Source: CAD feature listing. Evaluate the final solid. Frame: model axes, mm. Face numbers are marked on the shaded views. A direction names the side the tool comes from. Round coordinates to 2 decimals unless told otherwise and drop trailing zeros. Loops run counter-clockwise (first coordinate to the right, second up) from the corner with the lowest first, then second, coordinate; pieces in that order, holes last. Notation, with made-up numbers: M -25.5,17.5 L -16.5,17.5 A13 cw -16.5,23.5 Z; hole C 77.25,83 d10. An arc over 180 degrees is marked long. Answer as a JSON object with one key per item and string values.
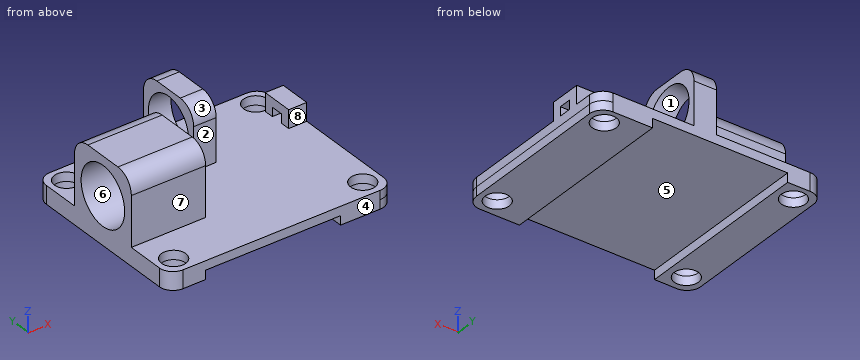
from build123d import *

# Parameters (mm, degrees)
CROQUIS1_W               = 49.8
CROQUIS1_H               = 39.8
CROQUIS1_R               = 2.7
SALIENTE_EXTRUIR1_DEPTH  = 6
CORTAR_EXTRUIR1_DEPTH    = 4
SALIENTE_EXTRUIR3_DEPTH  = 3
CROQUIS5_R               = 6.35
CORTAR_EXTRUIR2_DEPTH    = 3
SALIENTE_EXTRUIR4_DEPTH  = 10
SALIENTE_EXTRUIR5_DEPTH  = 2
CORTAR_EXTRUIR3_START    = -3
CORTAR_EXTRUIR3_DEPTH    = 3
CORTAR_EXTRUIR4_DEPTH    = 4
CROQUIS10_W              = 4
CROQUIS10_H              = 7
SALIENTE_EXTRUIR6_DEPTH  = 4
CORTAR_EXTRUIR5_START    = -4
CORTAR_EXTRUIR5_DEPTH    = 4
CROQUIS16_W              = 28.958796265
CROQUIS16_H              = 47.870649268
CORTAR_EXTRUIR6_DEPTH    = 2
CROQUIS17_W              = 5
CROQUIS17_H              = 16
CORTAR_EXTRUIR7_DEPTH    = 10
CORTAR_EXTRUIR8_DEPTH    = 2
SALIENTE_EXTRUIR7_DEPTH  = 2
CROQUIS22_R              = 6.5
SALIENTE_EXTRUIR9_DEPTH  = 15
SALIENTE_EXTRUIR10_DEPTH = 1.5
CROQUIS25_W              = 5
CROQUIS25_H              = 15
SALIENTE_EXTRUIR11_DEPTH = 13.5
CORTAR_EXTRUIR9_START    = -5
CROQUIS26_R              = 6
CORTAR_EXTRUIR9_DEPTH    = 5
REDONDEO2_R              = 4
CROQUIS27_W              = 8
CROQUIS27_H              = 39.8
CROQUIS27_R              = 2.7
CROQUIS27_W_2            = 11.8
SALIENTE_EXTRUIR13_DEPTH = 2
REDONDEO3_R              = 3


with BuildPart() as part:
    # Croquis1 → Saliente-Extruir1 (new body)
    with BuildSketch(Plane.XY):
        with Locations((-31.963412372, -3.757931034)):
            Rectangle(CROQUIS1_W, CROQUIS1_H)
        with Locations((-52.963412372, 12.342068966)):
            Circle(CROQUIS1_R, mode=Mode.SUBTRACT)
        with Locations((-10.963412372, 12.342068966)):
            Circle(CROQUIS1_R, mode=Mode.SUBTRACT)
        with Locations((-10.963412372, -19.657931034)):
            Circle(CROQUIS1_R, mode=Mode.SUBTRACT)
        with Locations((-52.963412372, -19.657931034)):
            Circle(CROQUIS1_R, mode=Mode.SUBTRACT)
    extrude(amount=SALIENTE_EXTRUIR1_DEPTH)

    # Croquis2 → Cortar-Extruir1 (cut)
    with BuildSketch(Plane.XY.offset(6)):
        with BuildLine():
            Line((-49.963412372, -16.757931034), (-13.963412372, -16.757931034))
            ThreePointArc((-13.963412372, -16.757931034), (-12.54919881, -16.172144597), (-11.963412372, -14.757931034))
            Line((-11.963412372, -14.757931034), (-11.963412372, 7.242068966))
            ThreePointArc((-11.963412372, 7.242068966), (-12.54919881, 8.656282528), (-13.963412372, 9.242068966))
            Line((-13.963412372, 9.242068966), (-49.963412372, 9.242068966))
            ThreePointArc((-49.963412372, 9.242068966), (-51.377625934, 8.656282528), (-51.963412372, 7.242068966))
            Line((-51.963412372, 7.242068966), (-51.963412372, -14.757931034))
            ThreePointArc((-51.963412372, -14.757931034), (-51.377625934, -16.172144597), (-49.963412372, -16.757931034))
        make_face()
    extrude(amount=-CORTAR_EXTRUIR1_DEPTH, mode=Mode.SUBTRACT)

    # Croquis4 → Saliente-Extruir3 (add)
    with BuildSketch(Plane(origin=(0, 0, 0), x_dir=(-1, 0, 0), z_dir=(0, 0, -1))):
        with BuildLine():
            Line((56.863412372, 4.242068966), (61.863412372, 4.242068966))
            Line((61.863412372, 4.242068966), (61.863412372, -0.257931034))
            Line((61.863412372, -0.257931034), (57.863412372, -0.257931034))
            ThreePointArc((57.863412372, -0.257931034), (57.358118834, -0.294597605), (56.863412372, -0.403829068))
            Line((56.863412372, -0.403829068), (56.863412372, 4.242068966))
        make_face()
        with BuildLine():
            Line((61.863412372, -11.757931034), (56.863412372, -11.757931034))
            Line((56.863412372, -11.757931034), (56.863412372, -7.112033001))
            ThreePointArc((56.863412372, -7.112033001), (57.358118834, -7.221264464), (57.863412372, -7.257931034))
            Line((57.863412372, -7.257931034), (61.863412372, -7.257931034))
            Line((61.863412372, -7.257931034), (61.863412372, -11.757931034))
        make_face()
    extrude(amount=-SALIENTE_EXTRUIR3_DEPTH)

    # Croquis5 → Cortar-Extruir2 (cut)
    with BuildSketch(Plane.XY.offset(3)):
        with Locations((-57.863412372, -3.757931034)):
            Circle(CROQUIS5_R)
    extrude(amount=CORTAR_EXTRUIR2_DEPTH, mode=Mode.SUBTRACT)

    # Croquis6 → Saliente-Extruir4 (add)
    with BuildSketch(Plane.XY.offset(3)):
        with BuildLine():
            Line((-61.863412372, 4.242068966), (-51.963412372, 4.242068966))
            Line((-51.963412372, 4.242068966), (-48.963412372, 4.242068966))
            Line((-48.963412372, 4.242068966), (-48.963412372, -11.757931034))
            Line((-48.963412372, -11.757931034), (-51.963412372, -11.757931034))
            Line((-51.963412372, -11.757931034), (-61.863412372, -11.757931034))
            Line((-61.863412372, -11.757931034), (-61.863412372, -8.689715701))
            ThreePointArc((-61.863412372, -8.689715701), (-51.513412372, -3.757931034), (-61.863412372, 1.173853632))
            Line((-61.863412372, 1.173853632), (-61.863412372, 4.242068966))
        make_face()
    extrude(amount=SALIENTE_EXTRUIR4_DEPTH)

    # Croquis7 → Saliente-Extruir5 (add)
    with BuildSketch(Plane.XY.offset(2)):
        Polygon((-51.963412372, -3.757931034), (-51.963412372, 4.242068966), (-48.963412372, 4.242068966), (-48.963412372, -11.757931034), (-51.963412372, -11.757931034), align=None)
    extrude(amount=SALIENTE_EXTRUIR5_DEPTH)

    # Croquis8 → Cortar-Extruir3 (cut)
    with BuildSketch(Plane.XY.offset(3).offset(CORTAR_EXTRUIR3_START)):
        with BuildLine():
            Line((-56.863412372, -0.403829068), (-56.863412372, -7.112033001))
            ThreePointArc((-56.863412372, -7.112033001), (-53.509310406, -3.757931034), (-56.863412372, -0.403829068))
        make_face()
    extrude(amount=CORTAR_EXTRUIR3_DEPTH, mode=Mode.SUBTRACT)

    # Croquis9 → Cortar-Extruir4 (cut)
    with BuildSketch(Plane.XY.offset(6)):
        Polygon((-56.863412372, -11.757931034), (-56.863412372, -27.492217147), (-1.817084798, -27.492217147), (-1.817084798, 22.861833321), (-56.863412372, 22.861833321), (-56.863412372, 4.242068966), (-47.172737702, 4.242068966), (-47.172737702, -11.757931034), align=None)
    extrude(amount=-CORTAR_EXTRUIR4_DEPTH, mode=Mode.SUBTRACT)

    # Croquis10 → Saliente-Extruir6 (add)
    with BuildSketch(Plane.XY.offset(2)):
        with Locations((-9.063412372, 5.842068966)):
            Rectangle(CROQUIS10_W, CROQUIS10_H)
    extrude(amount=SALIENTE_EXTRUIR6_DEPTH)

    # Croquis11 → Cortar-Extruir5 (cut)
    with BuildSketch(Plane(origin=(-7.063412372, 0, 0), x_dir=(0, 0, -1), z_dir=(1, 0, 0)).offset(CORTAR_EXTRUIR5_START)):
        Polygon((-2, 5.842068966), (-2, 7.242068966), (-4, 7.242068966), (-4, 4.442068966), (-2, 4.442068966), align=None)
    extrude(amount=CORTAR_EXTRUIR5_DEPTH, mode=Mode.SUBTRACT)

    # Croquis16 → Cortar-Extruir6 (cut)
    with BuildSketch(Plane.XY.offset(2)):
        with Locations((-49.718694927, -6.990346687)):
            Rectangle(CROQUIS16_W, CROQUIS16_H)
    extrude(amount=CORTAR_EXTRUIR6_DEPTH, mode=Mode.SUBTRACT)


with BuildPart() as cortar_extruir6_kept_piece:
    # of the separate pieces the step leaves, the one the design keeps (cortar_extruir6_pieces_kept)
    add(part.part.solids().sort_by_distance((-56.863412372, 16.142068966, 0))[0])

    # Croquis17 → Cortar-Extruir7 (cut)
    with BuildSketch(Plane.XY.offset(2)):
        with Locations((-59.363412372, -3.757931034)):
            Rectangle(CROQUIS17_W, CROQUIS17_H)
    extrude(amount=-CORTAR_EXTRUIR7_DEPTH, mode=Mode.SUBTRACT)

    # Croquis18 → Cortar-Extruir8 (cut)
    with BuildSketch(Plane.XY.offset(2)):
        with BuildLine():
            Line((-56.863412372, -0.403829068), (-50.513412372, -0.403829068))
            ThreePointArc((-50.513412372, -0.403829068), (-47.159310406, -3.757931034), (-50.513412372, -7.112033001))
            Line((-50.513412372, -7.112033001), (-56.863412372, -7.112033001))
            Line((-56.863412372, -7.112033001), (-56.863412372, -0.403829068))
        make_face()
    extrude(amount=-CORTAR_EXTRUIR8_DEPTH, mode=Mode.SUBTRACT)

    # Croquis20 → Saliente-Extruir7 (add)
    with BuildSketch(Plane.XY.offset(2)):
        with BuildLine():
            Line((-56.863412372, -0.403829068), (-56.863412372, -7.112033001))
            Line((-56.863412372, -7.112033001), (-50.513412372, -7.112033001))
            ThreePointArc((-50.513412372, -7.112033001), (-47.159310406, -3.757931034), (-50.513412372, -0.403829068))
            Line((-50.513412372, -0.403829068), (-56.863412372, -0.403829068))
        make_face()
    extrude(amount=-SALIENTE_EXTRUIR7_DEPTH)

    # Croquis22 → Saliente-Extruir9 (add)
    with BuildSketch(Plane.ZY.offset(56.863412372)):
        with BuildLine():
            Line((2, -3.757931034), (2, 4.742068966))
            Line((2, 4.742068966), (13, 4.742068966))
            ThreePointArc((13, 4.742068966), (15.828427125, 3.57049609), (17, 0.742068966))
            Line((17, 0.742068966), (17, -8.257931034))
            ThreePointArc((17, -8.257931034), (15.828427125, -11.086358159), (13, -12.257931034))
            Line((13, -12.257931034), (2, -12.257931034))
            Line((2, -12.257931034), (2, -3.757931034))
        make_face()
        with Locations(Location((8.55, -3.757931034, 0), (0, 0, 270))):
            Circle(CROQUIS22_R, mode=Mode.SUBTRACT)
    extrude(amount=-SALIENTE_EXTRUIR9_DEPTH)

    # Croquis23 → Saliente-Extruir10 (add)
    with BuildSketch(Plane(origin=(-41.863412372, 0, 0), x_dir=(0, 0, -1), z_dir=(1, 0, 0))):
        with BuildLine():
            Line((-13, -12.257931034), (-2, -12.257931034))
            Line((-2, -12.257931034), (-2, 4.742068966))
            Line((-2, 4.742068966), (-13, 4.742068966))
            ThreePointArc((-13, 4.742068966), (-15.828427125, 3.57049609), (-17, 0.742068966))
            Line((-17, 0.742068966), (-17, -8.257931034))
            ThreePointArc((-17, -8.257931034), (-15.828427125, -11.086358159), (-13, -12.257931034))
        make_face()
    extrude(amount=SALIENTE_EXTRUIR10_DEPTH)

    # Croquis25 → Saliente-Extruir11 (add)
    with BuildSketch(Plane.XY.offset(2)):
        with Locations((-30.563412372, 8.642068966)):
            Rectangle(CROQUIS25_W, CROQUIS25_H)
    extrude(amount=SALIENTE_EXTRUIR11_DEPTH)

    # Croquis26 → Cortar-Extruir9 (cut)
    with BuildSketch(Plane(origin=(-28.063412372, 0, 0), x_dir=(0, 0, -1), z_dir=(1, 0, 0)).offset(CORTAR_EXTRUIR9_START)):
        with Locations((-8.1, 8.642068966)):
            Circle(CROQUIS26_R)
    extrude(amount=CORTAR_EXTRUIR9_DEPTH, mode=Mode.SUBTRACT)

    # Redondeo2
    redondeo2_edges = [cortar_extruir6_kept_piece.edges().sort_by_distance(p)[0] for p in [
        (-30.563412372, 1.142068966, 15.5),
        (-30.563412372, 16.142068966, 15.5),
    ]]
    fillet(redondeo2_edges, radius=REDONDEO2_R)

    # Croquis27 → Saliente-Extruir13 (add)
    # profile 1 of 2: a face of its own
    with BuildSketch(Plane(origin=(0, 0, 0), x_dir=(-1, 0, 0), z_dir=(0, 0, -1))):
        with Locations((52.863412372, -3.757931034)):
            Rectangle(CROQUIS27_W, CROQUIS27_H)
        with Locations((52.963412372, -19.657931034)):
            Circle(CROQUIS27_R, mode=Mode.SUBTRACT)
        with Locations((52.963412372, 12.342068966)):
            Circle(CROQUIS27_R, mode=Mode.SUBTRACT)
    # profile 2 of 2: a face of its own
    with BuildSketch(Plane(origin=(0, 0, 0), x_dir=(-1, 0, 0), z_dir=(0, 0, -1))):
        with Locations((12.963412372, -3.757931034)):
            Rectangle(CROQUIS27_W_2, CROQUIS27_H)
        with Locations((10.963412372, 12.342068966)):
            Circle(CROQUIS27_R, mode=Mode.SUBTRACT)
        with Locations((10.963412372, -19.657931034)):
            Circle(CROQUIS27_R, mode=Mode.SUBTRACT)
    extrude(amount=SALIENTE_EXTRUIR13_DEPTH)

    # Redondeo3
    redondeo3_edges = [cortar_extruir6_kept_piece.edges().sort_by_distance(p)[0] for p in [
        (-56.863412372, 16.142068966, 0),
        (-7.063412372, 16.142068966, 0),
        (-7.063412372, -23.657931034, 0),
        (-56.863412372, -23.657931034, 0),
    ]]
    fillet(redondeo3_edges, radius=REDONDEO3_R)


solid = cortar_extruir6_kept_piece.part
Item 1: Access query for the marked faces 4, 5, 6, 7 and 8. Directions: +Z, -Z, +X, -X, +Y, -Y. A direction counts if a zero-diameter tool reaches every point of the face in a straight line with its end or side. Return the directions, or none.
Answer sheet:
{"face 4": "+Z, -Z, +X, -X, -Y", "face 5": "-Z, +Y, -Y", "face 6": "-X", "face 7": "+Z, +X, -X, -Y", "face 8": "+Z, +X, -Y"}
Item 2: Section D-D on x = -36. Return the cut outline in (y, z), then the cut area to 3 significant figures.
Answer sheet:
{"outline": "M -23.66,0 L 16.14,0 L 16.14,2 L -23.66,2 Z", "area": "79.6 mm²"}
Item 3: Pull-direction query (Z, two-part tool) for the marked faces 1, 2 and 3; classes: pulls with the +Z half, pulls with the -Z half, needs draft (parallel to the pull), parting line crosses it, or undercut.
Answer sheet:
{"face 1": "undercut", "face 2": "needs draft", "face 3": "pulls with the +Z half"}
Item 4: Contact query for flat-ended pins moving along their axis: pin 1 Ø1.2 at (x, z) = (-9.5, 4) entering from +Y; pin 2 Ø2 at (x, y) = (-22, -3.5) entering from -Z; pin 3 Ø1.2 at (x, z) = (-9, 3.5) entering from -Y. Output: stop coordinate, or through.
Answer sheet:
{"pin 1": "stops at y = 9.34", "pin 2": "stops at z = 0", "pin 3": "stops at y = 2.34"}
Item 5: Section A-A on y = -19. Return the cut outline in (x, z).
Answer sheet:
{"outline": "M -56.86,-2 L -55.58,-2 L -55.58,2 L -56.86,2 Z; M -50.34,-2 L -48.86,-2 L -48.86,0 L -18.86,0 L -18.86,-2 L -13.58,-2 L -13.58,2 L -50.34,2 Z; M -8.34,-2 L -7.06,-2 L -7.06,2 L -8.34,2 Z"}
Item 6: Line query: probe 1 along X at (y, z) = (1.5, 8); probe 2 along X at (y, z) = (3, 10.25); probe 3 along X at (y, z) = (4.5, 11.5). Output: solid intervals per line, ascending. Write a range as from..to.
Answer sheet:
{"probe 1": "x = -41.86..-40.36, -33.06..-28.06", "probe 2": "x = -56.86..-40.36, -33.06..-28.06", "probe 3": "x = -56.86..-40.36"}
Item 7: Section B-B on x = -51.5. Return the cut outline in (y, z).
Answer sheet:
{"outline": "M -23.66,-2 L -21.93,-2 L -21.93,2 L -23.66,2 Z; M -17.39,-2 L 10.07,-2 L 10.07,2 L 4.74,2 L 4.74,13 A4 ccw 0.74,17 L -8.26,17 A4 ccw -12.26,13 L -12.26,2 L -17.39,2 Z; M 14.61,-2 L 16.14,-2 L 16.14,2 L 14.61,2 Z; hole C -3.76,8.55 d13"}
Item 8: Section C-C on z = 7.5. Return the cut outline in (x, y).
Answer sheet:
{"outline": "M -56.86,-12.26 L -40.36,-12.26 L -40.36,4.74 L -56.86,4.74 L -56.86,2.66 L -41.86,2.66 L -41.86,-10.17 L -56.86,-10.17 Z; M -33.06,1.14 L -28.06,1.14 L -28.06,2.67 L -33.06,2.67 Z; M -33.06,14.61 L -28.06,14.61 L -28.06,16.14 L -33.06,16.14 Z"}
